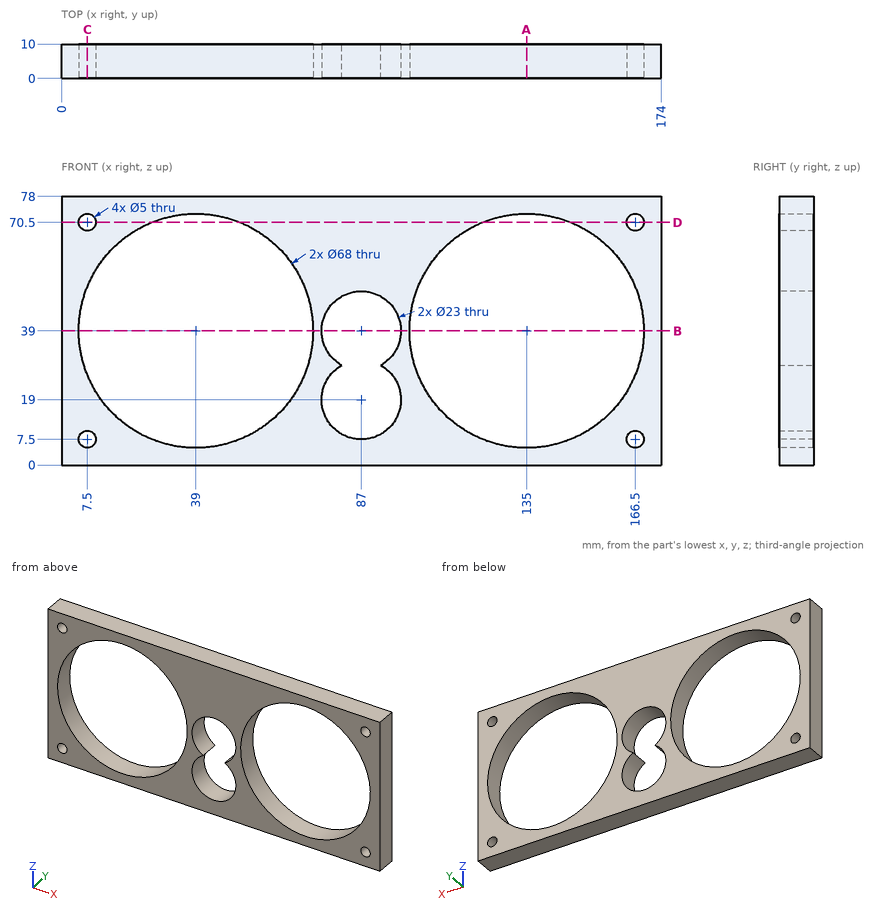
Study the drawing (mm; zero at the part's minimum x, y, z) and answer. Give positions to 0.01 mm unless a question says otherwise; leave off trailing zeros. Loops run counter-clockwise (first coordinate to the right, second up) from the corner with the lowest first, then second, coordinate; pieces in that order, holes last. Notation, with made-up numbers: (75, -36) -> (82, -36) arc R20 cw to (82, -25) -> close; hole circle Ø11 at (-14.5, 55). An arc over 180 degrees is marked (long way). Write item = value, one per line. Start each with the question number.
(1) Given pin 1 Ø2 at (x, y) = (28.5, 4.5) entering from -Z, flat-ended and moving along its own axis, determine where the tip first touches the part or whether it passes through.
(2) Find section C-C on x = 7.5. Give the vertices of the cut face in (y, z), and give its area (3 significant figures).
(3) Find section B-B on z = 39. Give the vertices of the cut face in (x, y).
(4) Find section D-D on z = 70.5. Give the vertices of the cut face in (x, y), and give its area (3 significant figures).
(5) Find section A-A on x = 135. Give the vertices of the cut face in (y, z), and give its area (3 significant figures).
(6) Find the intervals of material crossed by probe 1 along X at (y, z) = (3.75, 39); probe 2 along X at (y, z) = (1.5, 45.5); probe 3 along X at (y, z) = (5.5, 64.5), in increasing order. Write a range as from..to.
From the geometry:
q1.pin_1 = 0
q2.outline = (0, 0) -> (10, 0) -> (10, 5) -> (0, 5) -> close; (0, 10) -> (10, 10) -> (10, 26.2) -> (0, 26.2) -> close; (0, 51.8) -> (10, 51.8) -> (10, 68) -> (0, 68) -> close; (0, 73) -> (10, 73) -> (10, 78) -> (0, 78) -> close
q2.area = 424 mm^2
q3.outline = (0, 0) -> (5, 0) -> (5, 10) -> (0, 10) -> close; (73, 0) -> (75.5, 0) -> (75.5, 10) -> (73, 10) -> close; (98.5, 0) -> (101, 0) -> (101, 10) -> (98.5, 10) -> close; (169, 0) -> (174, 0) -> (174, 10) -> (169, 10) -> close
q4.outline = (0, 0) -> (5, 0) -> (5, 10) -> (0, 10) -> close; (10, 0) -> (26.2, 0) -> (26.2, 10) -> (10, 10) -> close; (51.8, 0) -> (122.2, 0) -> (122.2, 10) -> (51.8, 10) -> close; (147.8, 0) -> (164, 0) -> (164, 10) -> (147.8, 10) -> close; (169, 0) -> (174, 0) -> (174, 10) -> (169, 10) -> close
q4.area = 1,130 mm^2
q5.outline = (0, 0) -> (10, 0) -> (10, 5) -> (0, 5) -> close; (0, 73) -> (10, 73) -> (10, 78) -> (0, 78) -> close
q5.area = 100 mm^2
q6.probe_1 = 0..5, 73..75.5, 98.5..101, 169..174
q6.probe_2 = 0..5.63, 72.37..77.51, 96.49..101.63, 168.37..174
q6.probe_3 = 0..16.51, 61.49..112.51, 157.49..174
